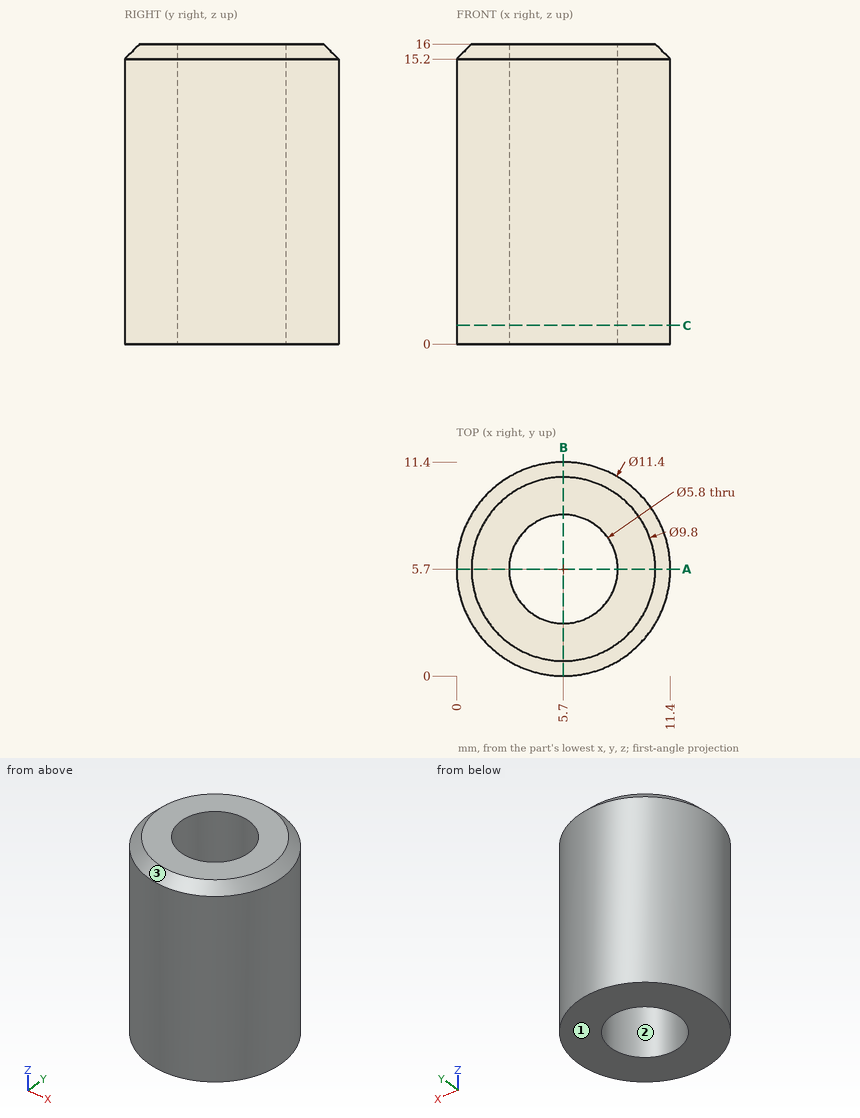
The figure shows three views and two pictorial views of one solid part (mm, origin at its lowest corner). Answer the questions. Coordinates: 2 decimals unless noted, no trailing zeros. Loops run counter-clockwise (first coordinate to the right, second up) from the corner with the lowest first, then second, coordinate; pieces in that order, holes last.
1) Find section A-A on y = 5.7. Write down the section's boundary in (x, z).
2) Determine the mould class of the marked faces 1, 2 and 3 for opening direction Y: pulls with the +Y half, pulls with the -Y half, needs draft (parallel to the pull), parting line crosses it, or undercut.
3) Find the intervals of material crossed by L1, parallel to Y at x = 5.7, z = 7; L2, parallel to Y at x = 6.25, z = 12.5, in increasing order.
4) Flat-ended cylindrical pins translate along their axes: pin 1 Ø3 at (y, z) = (1.5, 9) entering from +X; pin 2 Ø1 at (y, z) = (1.5, 13) entering from -X; pin 3 Ø2 at (y, z) = (1.5, 7.5) entering from +X. Find the tip coordinate at first contact, or state that the pin passes through.
5) Find section C-C on z = 1. Write down the section's boundary in (x, y).
Values:
1. outline: (0, 0) - (2.8, 0) - (2.8, 16) - (0.8, 16) - (0, 15.2) - close; (8.6, 0) - (11.4, 0) - (11.4, 15.2) - (10.6, 16) - (8.6, 16) - close
2. face 1: needs draft
2. face 2: undercut
2. face 3: parting line crosses it
3. L1: y = 0 to 2.8, 8.6 to 11.4
3. L2: y = 0.03 to 2.85, 8.55 to 11.37
4. pin 1: stops at x = 10.72
4. pin 2: stops at x = 1.36
4. pin 3: stops at x = 10.42
5. outline: circle Ø11.4 at (5.7, 5.7); hole circle Ø5.8 at (5.7, 5.7)
